```python
from build123d import *

# Parameters (mm, degrees)
BOSS_EXTRUDE1_DEPTH                                 = 4
BOSS_EXTRUDE1_DEPTH_BACK                            = 2
SKETCH1_R                                           = 17.5
SKETCH1_R_2                                         = 11.6
BOSS_EXTRUDE2_DEPTH                                 = 6
CSK_FOR_M5_COUNTERSUNK_FLAT_HEAD_SCREW2_D           = 5.5
CSK_FOR_M5_COUNTERSUNK_FLAT_HEAD_SCREW2_CSINK_D     = 10.4
CSK_FOR_M5_COUNTERSUNK_FLAT_HEAD_SCREW2_CSINK_ANGLE = 90
FILLET1_R                                           = 3
SKETCH5_R                                           = 11.6
SKETCH5_R_2                                         = 10
BOSS_EXTRUDE3_DEPTH                                 = 2


with BuildPart() as part:
    # Sketch1 → Boss-Extrude1 (new, two sides: drawn at the far end of the back side and taken through both)
    with BuildSketch(Plane(origin=(0, 0, 0), x_dir=(0, 0, -1), z_dir=(1, 0, 0)).offset(-BOSS_EXTRUDE1_DEPTH_BACK)):
        Circle(SKETCH1_R)
        Circle(SKETCH1_R_2, mode=Mode.SUBTRACT)
    extrude(amount=BOSS_EXTRUDE1_DEPTH + BOSS_EXTRUDE1_DEPTH_BACK)

    # Sketch2 → Boss-Extrude2 (add)
    with BuildSketch(Plane.ZY.offset(2)):
        with BuildLine():
            Line((-8.736495138, 15.163233584), (-38.275718713, 39.949585191))
            ThreePointArc((-38.275718713, 39.949585191), (-46.72871103, 39.210044191), (-45.98917003, 30.757051874))
            Line((-45.98917003, 30.757051874), (-16.449946454, 5.970700266))
            ThreePointArc((-16.449946454, 5.970700266), (-15.159340579, 8.743248436), (-13.405777755, 11.24878317))
            ThreePointArc((-13.405777755, 11.24878317), (-11.242810713, 13.410786975), (-8.736495138, 15.163233584))
        make_face()
        with BuildLine():
            Line((-6, 32), (-6, 16.439282223))
            ThreePointArc((-6, 16.439282223), (-3.046519416, 17.232780375), (0, 17.5))
            ThreePointArc((0, 17.5), (3.046519416, 17.232780375), (6, 16.439282223))
            Line((6, 16.439282223), (6, 32))
            ThreePointArc((6, 32), (0, 38), (-6, 32))
        make_face()
    extrude(amount=-BOSS_EXTRUDE2_DEPTH)

    # CSK for M5 Countersunk Flat Head Screw2 (through all)
    with Locations(Plane.ZY.offset(2)):
        with Locations((0, 32), (-42.132444372, 35.353318533)):
            CounterSinkHole(CSK_FOR_M5_COUNTERSUNK_FLAT_HEAD_SCREW2_D / 2, CSK_FOR_M5_COUNTERSUNK_FLAT_HEAD_SCREW2_CSINK_D / 2, counter_sink_angle=CSK_FOR_M5_COUNTERSUNK_FLAT_HEAD_SCREW2_CSINK_ANGLE)

    # Fillet1
    # the kernel refuses this fillet: 3 mm, written as the material it adds along each edge
    with BuildSketch(Plane(origin=(-2, 5.970700266, -16.449946454), x_dir=(0, -0.9565409410444833, -0.2915980591597522), z_dir=(1, 0, 0)), Plane(origin=(4, 15.163233584, -8.736495138), x_dir=(0, 0.45326962070001187, 0.8913734632299009), z_dir=(-1, 0, 0)), Plane(origin=(-2, 16.439282223, -6), x_dir=(0, -0.3914755922176966, -0.9201884919394524), z_dir=(1, 0, 0)), Plane(origin=(4, 16.439282223, 6), x_dir=(0, -0.39147559221769407, 0.9201884919394534), z_dir=(-1, 0, 0))) as fillet1_piece_1:
        with BuildLine():
            CenterArc((1.985655892, 2.995901464), FILLET1_R, 203.046346261, 63.958350044)
            Line((-0.774909584, 1.821474687), (0, 0))
            ThreePointArc((0, 0), (0.914446792, 0.02390813), (1.828893584, 0))
        make_face()
    extrude(amount=6)

    # Sketch5 → Boss-Extrude3 (add)
    with BuildSketch(Plane.ZY.offset(2)):
        with Locations(Location((0, 0, 0), (0, 0, 180))):
            Circle(SKETCH5_R)
        Circle(SKETCH5_R_2, mode=Mode.SUBTRACT)
    extrude(amount=-BOSS_EXTRUDE3_DEPTH)


solid = part.part
```
Check sheet for the modelled part. Datum: model origin and axes. Units: mm. A direction names the side the tool comes from. Round coordinates to 2 decimals unless told otherwise and drop trailing zeros. Loops run counter-clockwise (first coordinate to the right, second up) from the corner with the lowest first, then second, coordinate; pieces in that order, holes last. Notation, with made-up numbers: (-18, 36) - (21, 36) arc R15 cw to (21, 46) - close; hole circle Ø1 at (-6.75, 76). An arc over 180 degrees is marked (long way). Write item = value, one per line. Start each with the question number.
Q1. Release check for a two-part mould opening along Z. For faces 1 (the face through (0, -10, -3)), 2 (the face through (2.25, 34.727, 0.358)), 3 (the face through (0.958, 39.31, -46.643)), 4 (the face through (4, 12, -14)) record: pulls with the +Z half, pulls with the -Z half, needs draft (parallel to the pull), parting line crosses it, or undercut.
Q2. Section check C-C (x = 2.05). Record the boundary of the cut face in (y, z), plus the area to 3 significant figures.
Q3. Section check B-B (z = 0). Record the boundary of the cut face in (x, y).
Q4. Depth check by flat-ended pin: P1, Ø3, axis at x = 1, z = -39, coming from the +Y side; P2, Ø6.5, axis at y = 32, z = 0, coming from the -X side; P3, Ø2, axis at x = 3.5, z = -39.5, coming from the -Y side. Enter the tip coordinate at first touch or a pass-through.
Q5. Section check D-D (y = 24). Record the boundary of the cut face in (x, z).
Q6. Section check A-A (y = 0). Record the boundary of the cut face in (x, z).
Q7. Thickness scan on L1, parallel to Y at x = 2.4, z = 0; L2, parallel to Y at x = -0.85, z = 0; L3, parallel to Z at x = 2.5, y = 32. Record the ranges inside material, lowest first.
Q8. Access from +Z, -Z, +X, -X, +Y, -Y to the whole of each face (thin tool, end or side, straight path). Record for faces 5 (the face through (0.96, -15.62, 7.89)), 6 (the face through (0.96, 16.99, -6.36)), 7 (the face through (1.97, 0.51, 11.59)), 8 (the face through (0.33, 32.55, -41.51)), 9 (the face through (1, 25, 6)).
Derived:
q1.face_1 = undercut
q1.face_2 = undercut
q1.face_3 = parting line crosses it
q1.face_4 = needs draft
q2.outline = (4.22, -16.98) arc R3 cw to (7.24, -17.97) - (30.76, -45.99) arc R6 ccw to (39.95, -38.28) - (16.44, -10.25) arc R3 cw to (15.88, -7.4) arc R3 cw to (18.42, -6) - (32, -6) arc R6 ccw to (32, 6) - (18.42, 6) arc R3 cw to (15.72, 7.68) arc R17.5 ccw (long way) to start; hole circle Ø23.2 at (0, 0); hole circle Ø5.5 at (32, 0); hole circle Ø5.5 at (35.35, -42.13)
q2.area = 1,240 mm^2
q3.outline = (-2, -17.5) - (4, -17.5) - (4, -11.6) - (0, -11.6) - (0, -10) - (-2, -10) - close; (-2, 10) - (0, 10) - (0, 11.6) - (4, 11.6) - (4, 29.25) - (0.45, 29.25) - (-2, 26.8) - close; (-2, 37.2) - (0.45, 34.75) - (4, 34.75) - (4, 38) - (-2, 38) - close
q4.P1 = 41.13
q4.P2 = -0.05
q4.P3 = 24.47
q5.outline = (-2, -37.94) - (4, -37.94) - (4, -19.27) - (-2, -19.27) - close; (-2, -6) - (4, -6) - (4, 6) - (-2, 6) - close
q6.outline = (-2, -17.5) - (4, -17.5) - (4, -11.6) - (0, -11.6) - (0, -10) - (-2, -10) - close; (-2, 10) - (0, 10) - (0, 11.6) - (4, 11.6) - (4, 17.5) - (-2, 17.5) - close
q7.L1 = -17.5 to -11.6, 11.6 to 29.25, 34.75 to 38
q7.L2 = -17.5 to -10, 10 to 27.95, 36.05 to 38
q7.L3 = -47.11 to -28.8, -6 to -2.75, 2.75 to 6
q8.face_5 = +X, -X
q8.face_6 = +X, -X, +Y
q8.face_7 = +X
q8.face_8 = -X
q8.face_9 = +Z, +X, -X, +Y
